```python
from build123d import *

# Parameters (mm, degrees)
SKETCH1_W           = 40
SKETCH1_H           = 30
BOSS_EXTRUDE1_DEPTH = 10
SKETCH5_W           = 40
SKETCH5_H           = 27
BOSS_EXTRUDE2_DEPTH = 3
SKETCH2_W           = 11.666666667
SKETCH2_H           = 27
SKETCH2_W_2         = 11.666666666
CUT_EXTRUDE1_DEPTH  = 11
SKETCH4_W           = 6
SKETCH4_H           = 3
CUT_EXTRUDE2_DEPTH  = 8
SKETCH6_W           = 19.333333334
SKETCH6_H           = 16
CUT_EXTRUDE3_DEPTH  = 2
CHAMFER2_SIZE       = 3
BOSS_EXTRUDE3_DEPTH = 2
SKETCH9_R           = 1.5
CUT_EXTRUDE5_DEPTH  = 2
SKETCH11_W          = 40
SKETCH11_H          = 30
CUT_EXTRUDE6_DEPTH  = 1
CHAMFER3_SIZE       = 2
SKETCH14_W          = 6
SKETCH14_H          = 2
BOSS_EXTRUDE4_DEPTH = 4
SKETCH15_R          = 1.5
CUT_EXTRUDE7_DEPTH  = 4
CHAMFER7_SIZE       = 4
SKETCH16_W          = 13.666666666
SKETCH16_H          = 6.5
CUT_EXTRUDE8_DEPTH  = 3


with BuildPart() as part:
    # Sketch1 → Boss-Extrude1 (new body)
    with BuildSketch(Plane(origin=(0, 0, 0), x_dir=(1, 0, 0), z_dir=(0, 1, 0))):
        Rectangle(SKETCH1_W, SKETCH1_H)
    extrude(amount=BOSS_EXTRUDE1_DEPTH)

    # Sketch5 → Boss-Extrude2 (add)
    with BuildSketch(Plane(origin=(0, 10, 0), x_dir=(1, 0, 0), z_dir=(0, 1, 0))):
        with Locations((0, -1.5)):
            Rectangle(SKETCH5_W, SKETCH5_H)
    extrude(amount=BOSS_EXTRUDE2_DEPTH)

    # Sketch2 → Cut-Extrude1 (cut)
    with BuildSketch(Plane(origin=(0, 13, 0), x_dir=(1, 0, 0), z_dir=(0, 1, 0))):
        with Locations((-12.666666666, 1.5)):
            Rectangle(SKETCH2_W, SKETCH2_H)
        with Locations((0, 1.5)):
            Rectangle(SKETCH2_W_2, SKETCH2_H)
        with Locations((12.666666666, 1.5)):
            Rectangle(SKETCH2_W, SKETCH2_H)
    extrude(amount=-CUT_EXTRUDE1_DEPTH, mode=Mode.SUBTRACT)

    # Sketch4 → Cut-Extrude2 (cut)
    with BuildSketch(Plane(origin=(0, 13, 0), x_dir=(1, 0, 0), z_dir=(0, 1, 0))):
        with Locations((-12.666666667, -13.5)):
            Rectangle(SKETCH4_W, SKETCH4_H)
        with Locations((0, -13.5)):
            Rectangle(SKETCH4_W, SKETCH4_H)
        with Locations((12.666666667, -13.5)):
            Rectangle(SKETCH4_W, SKETCH4_H)
    extrude(amount=-CUT_EXTRUDE2_DEPTH, mode=Mode.SUBTRACT)

    # Sketch6 → Cut-Extrude3 (cut)
    with BuildSketch(Plane(origin=(0, 13, 0), x_dir=(1, 0, 0), z_dir=(0, 1, 0))):
        with Locations((0, -7)):
            Rectangle(SKETCH6_W, SKETCH6_H)
    extrude(amount=-CUT_EXTRUDE3_DEPTH, mode=Mode.SUBTRACT)

    # Chamfer2
    chamfer2_edges = [part.edges().sort_by_distance(p)[0] for p in [
        (19.25, 10, -12),
        (6.333333333, 10, -12),
        (-6.333333333, 10, -12),
        (-19.25, 10, -12),
    ]]
    chamfer(chamfer2_edges, length=CHAMFER2_SIZE - 0.0001)  # a hair under: the kernel refuses the full size

    # Sketch8 → Boss-Extrude3 (add)
    with BuildSketch(Plane(origin=(0, 13, 0), x_dir=(1, 0, 0), z_dir=(0, 1, 0))):
        Polygon((20, -10), (27.39103626, -13.061467459), (24.712252234, -19.528624186), (15.666666667, -15.781819965), (15.666666667, -15), (18.5, -12), align=None)
    boss_extrude3 = extrude(amount=-BOSS_EXTRUDE3_DEPTH)

    # Mirror1: Boss-Extrude3 across plane
    add(boss_extrude3.mirror(Plane(origin=(0, 0, 0), x_dir=(0, 0, 1), z_dir=(1, 0, 0))))

    # Sketch9 → Cut-Extrude5 (cut)
    with BuildSketch(Plane.XZ.offset(-11)):
        with Locations(Location((-22.5, 14.5, 0), (0, 0, 270))):
            Circle(SKETCH9_R)
        with Locations(Location((22.5, 14.5, 0), (0, 0, 270))):
            Circle(SKETCH9_R)
    extrude(amount=-CUT_EXTRUDE5_DEPTH, mode=Mode.SUBTRACT)

    # Sketch11 → Cut-Extrude6 (cut)
    with BuildSketch(Plane.XZ):
        Rectangle(SKETCH11_W, SKETCH11_H)
    extrude(amount=-CUT_EXTRUDE6_DEPTH, mode=Mode.SUBTRACT)

    # Chamfer3
    chamfer3_edges = [part.edges().sort_by_distance(p)[0] for p in [
        (20, 6, 15),
        (-20, 6, 15),
        (0, 1, 15),
    ]]
    chamfer(chamfer3_edges, length=CHAMFER3_SIZE)

    # Sketch14 → Boss-Extrude4 (add)
    with BuildSketch(Plane.XZ.offset(-1)):
        with Locations((0, -14)):
            Rectangle(SKETCH14_W, SKETCH14_H)
    extrude(amount=BOSS_EXTRUDE4_DEPTH)

    # Sketch15 → Cut-Extrude7 (cut)
    with BuildSketch(Plane(origin=(0, 0, -15), x_dir=(-1, 0, 0), z_dir=(0, 0, -1))):
        with Locations((0, -0.5)):
            Circle(SKETCH15_R)
    extrude(amount=-CUT_EXTRUDE7_DEPTH, mode=Mode.SUBTRACT)

    # Chamfer7
    chamfer7_edges = [part.edges().sort_by_distance(p)[0] for p in [
        (3, 1, -14),
        (-3, 1, -14),
    ]]
    chamfer(chamfer7_edges, length=CHAMFER7_SIZE - 0.0001)  # a hair under: the kernel refuses the full size

    # Sketch16 → Cut-Extrude8 (cut)
    with BuildSketch(Plane(origin=(0, 13, 0), x_dir=(1, 0, 0), z_dir=(0, 1, 0))):
        with Locations((0, 11.75)):
            Rectangle(SKETCH16_W, SKETCH16_H)
    extrude(amount=-CUT_EXTRUDE8_DEPTH, mode=Mode.SUBTRACT)


solid = part.part
```
Work out the finished part from the listing and answer in its coordinate system (mm). A direction names the side the tool comes from. Round coordinates to 2 decimals unless told otherwise and drop trailing zeros. Write each loop counter-clockwise with the first axis right and the second up, starting at its lowest first coordinate (ties: lowest second). Pieces come first, ordered by that corner, then holes.
1) A cutting plane is placed at C-C on z = -10. Determine the outline of the cut face in (x, y).
2) A cutting plane is placed at B-B on x = -22.5. Determine the outline of the cut face in (y, z), and give its area (3 significant figures).
3) Consider probe 1 along X at (y, z) = (11, -3); probe 2 along X at (y, z) = (11.7, 14.5); probe 3 along Y at (x, z) = (0, -13.6). Determine where each line is inside the solid, lowest interval first.
4) A cutting plane is placed at A-A on y = -0.5. Determine the outline of the cut face in (x, z).
5) Which of the six approach directions +Z, -Z, +X, -X, +Y, -Y give full straight-line access (tool end or side, diameter ignored) to faces 4 (the face through (0, 4, 15)), 5 (the face through (-15.667, 9, 13)), 6 (the face through (-19, 6, 14)), 7 (the face through (-13, 4, 12))?
6) Flat-ended cylindrical pins translate along their axes: P1, Ø5, axis at x = 8, z = -5, coming from the -Y side; P2, Ø0.9, axis at x = -12, z = 13.5, coming from the +Y side; P3, Ø8, axis at x = 10.5, z = 9, coming from the +Y side. Find the tip coordinate at first contact, or state that the pin passes through.
7) A cutting plane is placed at D-D on x = -12.5. Determine the outline of the cut face in (y, z).
8) Determine the mould class of faces 1 (the face through (6.833, 6, -1)), 2 (the face through (23.51, 11.99, 15.61)), 3 (the face through (13, 4, 12)) for opening direction Z: pulls with the +Z half, pulls with the -Z half, needs draft (parallel to the pull), parting line crosses it, or undercut.
Entries:
1. outline: (-20, 1) - (20, 1) - (20, 13) - (18.5, 13) - (18.5, 2) - (6.83, 2) - (6.83, 10) - (5.83, 10) - (5.83, 2) - (-5.83, 2) - (-5.83, 10) - (-6.83, 10) - (-6.83, 2) - (-18.5, 2) - (-18.5, 13) - (-20, 13) - close
2. outline: (11, 11.04) - (13, 11.04) - (13, 13) - (11, 13) - close; (11, 16) - (13, 16) - (13, 18.61) - (11, 18.61) - close
2. area: 9.15 mm2
3. probe 1: x = -20 to -18.5, -6.83 to -5.83, 5.83 to 6.83, 18.5 to 20
3. probe 2: x = -26.8 to -24, -21 to -15.67, 15.67 to 21, 24 to 26.8
3. probe 3: y = -3 to -2, 1 to 2
4. outline: (-5.5, -15) - (-1.5, -15) - (-1.5, -13) - (-5.5, -13) - close; (1.5, -15) - (5.5, -15) - (5.5, -13) - (1.5, -13) - close
5. face 4: +Z, +X, -X, -Y
5. face 5: +Z, -Z, +Y
5. face 6: +Z, -X, -Y
5. face 7: -Z, +Y
6. P1: stops at y = 1
6. P2: stops at y = 5
6. P3: stops at y = 11
7. outline: (1, -15) - (2, -15) - (2, 12) - (5, 12) - (5, 15) - (3, 15) - (1, 13) - close
8. face 1: needs draft
8. face 2: undercut
8. face 3: pulls with the -Z half
